Here's the drawing with two shaded views (mm, measured from the low corner). I have some questions. Give positions to 0.01 mm unless a question says otherwise; leave off trailing zeros. Loops run counter-clockwise (first coordinate to the right, second up) from the corner with the lowest first, then second, coordinate; pieces in that order, holes last. Notation, with made-up numbers: (39, 62) - (96, 62) arc R7 cw to (96, 75) - close; hole circle Ø2 at (55, 60). An arc over 180 degrees is marked (long way). Use one line per item in the form item = value.
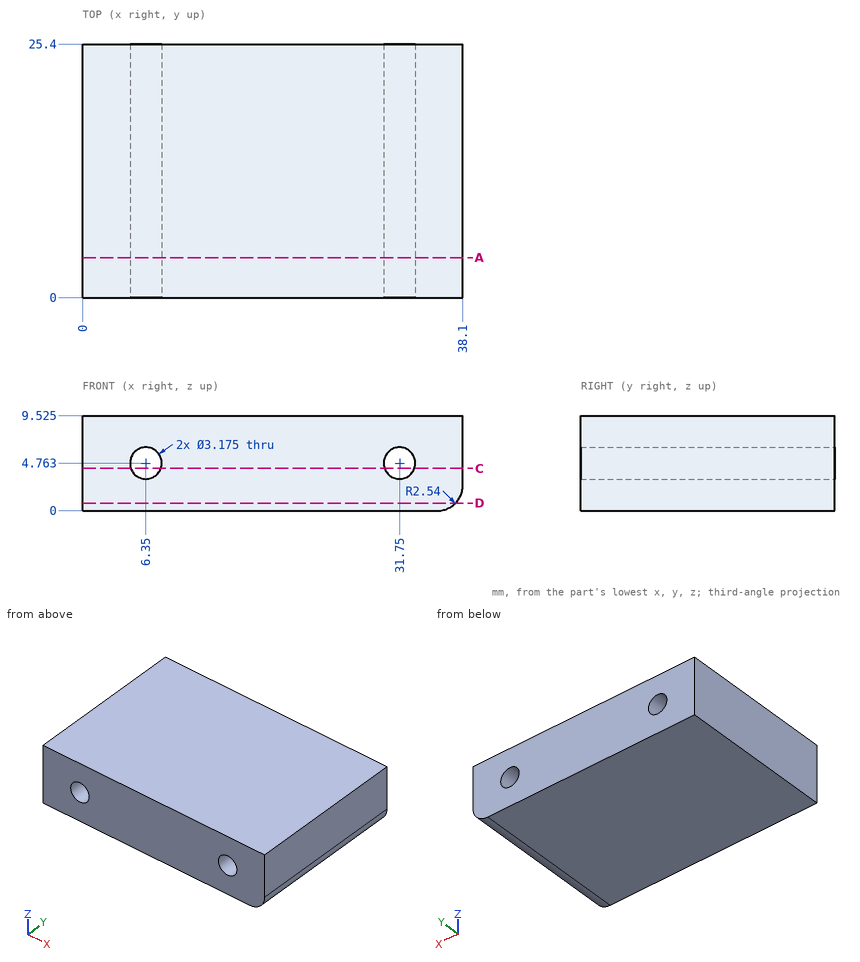
(1) If we section it at D-D (z = 0.75): List the corners of the cut face in (x, y) for me.
Geometry says:
outline = (0, 0) - (37.36, 0) - (37.36, 25.4) - (0, 25.4) - close
(2) For P1, Ø1.9, axis at x = 31.75, z = 4.76, coming from the -Y side, with a flat end and sliding along its axis, tell me the tip position at first contact or that it passes through.
Geometry says:
P1 = through
(3) If we section it at A-A (y = 4): Give the number of separate pieces and of enclosed holes in the cut face, plus the area to 3 significant figures.
Geometry says:
separate_pieces = 1
enclosed_holes = 2
area = 346 mm²
(4) If I drill on probe 1 along X at (y, z) = (14.5, 4.25); probe 2 along X at (y, z) = (3, 3.75) (1 decimal); probe 3 along Z at (x, y) = (5, 6) (1 decimal), over which ranges is the centre line in solid material (lowest first)?
Geometry says:
probe_1 = 0 to 4.85, 7.85 to 30.25, 33.25 to 38.1
probe_2 = 0 to 5.1, 7.6 to 30.5, 33 to 38.1
probe_3 = 0 to 3.9, 5.6 to 9.5
(5) If we section it at C-C (z = 4.25): List the corners of the cut face in (x, y) for me, plus the area to 3 significant figures.
Geometry says:
outline = (0, 0) - (4.85, 0) - (4.85, 25.4) - (0, 25.4) - close; (7.85, 0) - (30.25, 0) - (30.25, 25.4) - (7.85, 25.4) - close; (33.25, 0) - (38.1, 0) - (38.1, 25.4) - (33.25, 25.4) - close
area = 815 mm²
